CAD build for the part. Positions are in the model's coordinates, mm. Face numbers are marked on the shaded views. A direction names the side the tool comes from. Coordinates: 2 decimals unless noted, no trailing zeros. Order: outer loops, then holes, each group sorted by start corner. A loop starts at its lowest first (then second) coordinate and runs counter-clockwise, first axis right, second up. Notation, with made-up numbers: (55, 14) - (67, 14) arc R25 cw to (67, 35) - close; hole circle Ø4 at (51.5, 36.5). An arc over 180 degrees is marked (long way). Use one line per item in the form item = value.
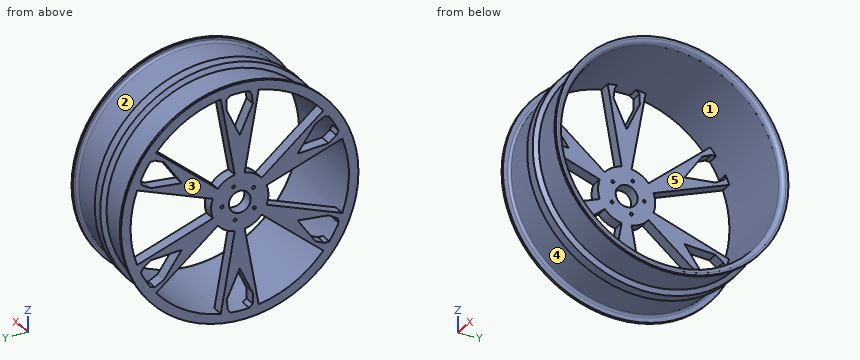
```python
from build123d import *

# Parameters (mm, degrees)
F2_R     = 3.1146523594
F2_R_2   = 22.9197931693
F3_DEPTH = 25
F4_COUNT = 6
F5_DEPTH = 25


# Not quite as in the source:
# - a feature names something its author has since deleted; it is built from what else it names


with BuildPart() as f1:
    # F0 (on Top) → F1 (revolve)
    with BuildSketch(Plane.XY):
        with BuildLine():
            Line((-79.7097083151, 53.5523933172), (-79.7097083151, 33.5523933172))
            Line((-79.7097083151, 33.5523933172), (113.4902916849, 33.5523933172))
            ThreePointArc((113.4902916849, 33.5523933172), (120.5613594967, 36.4813255054), (123.4902916849, 43.5523933172))
            Line((123.4902916849, 43.5523933172), (123.4902916849, 48.5523933172))
            Line((123.4902916849, 48.5523933172), (118.4902916849, 48.5523933172))
            Line((118.4902916849, 48.5523933172), (118.4902916849, 43.5523933172))
            ThreePointArc((118.4902916849, 43.5523933172), (117.0258255908, 40.0168594113), (113.4902916849, 38.5523933172))
            Line((113.4902916849, 38.5523933172), (38.4902916849, 38.5523933172))
            Line((38.4902916849, 38.5523933172), (5.2902916849, 38.5523933172))
            Line((5.2902916849, 38.5523933172), (-69.7097083151, 38.5523933172))
            ThreePointArc((-69.7097083151, 38.5523933172), (-73.2452422211, 40.0168594113), (-74.7097083151, 43.5523933172))
            Line((-74.7097083151, 43.5523933172), (-74.7097083151, 53.5523933172))
            Line((-74.7097083151, 53.5523933172), (-79.7097083151, 53.5523933172))
        make_face()
        Polygon((11.0637943768, 48.5523933172), (5.2902916849, 38.5523933172), (38.4902916849, 38.5523933172), (32.716788993, 48.5523933172), align=None)
    revolve(axis=Axis((21.8902916849, -195.0476066828, 0), (1, 0, 0)))

    # F2 (on face) → F3 (join)
    with BuildSketch(Plane(origin=(-79.7097083151, 0, 0), x_dir=(0, -1, 0), z_dir=(-1, 0, 0))):
        with BuildLine():
            ThreePointArc((184.6287160228, 59.0884651807), (189.8182621179, 59.7716818855), (195.0476066828, 60))
            Line((195.0476066828, 60), (195.0476066828, 139.9987626345))
            Line((195.0476066828, 139.9987626345), (167.5774196696, 198.9087687919))
            Line((167.5774196696, 198.9087687919), (167.7933331286, 221.202246743))
            Line((167.7933331286, 221.202246743), (175.3516332681, 227.7499256449))
            ThreePointArc((175.3516332681, 227.7499256449), (165.3226894728, 226.6591919532), (155.3516332681, 225.1270523386))
            Line((155.3516332681, 225.1270523386), (184.6287160228, 59.0884651807))
        make_face()
        with BuildLine():
            Line((195.0476066828, 139.9987626345), (195.0476066828, 60))
            ThreePointArc((195.0476066828, 60), (200.2769512476, 59.7716818855), (205.4664973428, 59.0884651807))
            Line((205.4664973428, 59.0884651807), (234.7435800974, 225.1270523386))
            ThreePointArc((234.7435800974, 225.1270523386), (224.7725238927, 226.6591919532), (214.7435800974, 227.7499256449))
            Line((214.7435800974, 227.7499256449), (220.1414219841, 219.3318912564))
            Line((220.1414219841, 219.3318912564), (222.5177936959, 198.9087687919))
            Line((222.5177936959, 198.9087687919), (195.0476066828, 139.9987626345))
        make_face()
        with BuildLine():
            ThreePointArc((205.4664973428, 59.0884651807), (200.2769512476, 59.7716818855), (195.0476066828, 60))
            ThreePointArc((195.0476066828, 60), (189.8182621179, 59.7716818855), (184.6287160228, 59.0884651807))
            ThreePointArc((184.6287160228, 59.0884651807), (156.4803501016, -45.9626665871), (255.0476066828, 0))
            ThreePointArc((255.0476066828, 0), (241.0102732699, 38.5672565812), (205.4664973428, 59.0884651807))
        make_face()
        with Locations((158.1552479456, -1.5052259386)):
            Circle(F2_R, mode=Mode.SUBTRACT)
        with Locations((185.0787958079, -35.5518585739)):
            Circle(F2_R, mode=Mode.SUBTRACT)
        with Locations((195.0476066828, 0)):
            Circle(F2_R_2, mode=Mode.SUBTRACT)
        with Locations((225.7789014718, -20.4670310233)):
            Circle(F2_R, mode=Mode.SUBTRACT)
        with Locations((224.0094022556, 22.9025377527)):
            Circle(F2_R, mode=Mode.SUBTRACT)
        with Locations((182.215685933, 34.6215777831)):
            Circle(F2_R, mode=Mode.SUBTRACT)
    extrude(amount=-F3_DEPTH)

    # F4: F1 ×6 about axis
    f4_axis = Axis((21.8902916849, -195.0476066828, 0), (1, 0, 0))


with BuildPart() as f1_1:
    add(f1.part)
    for i in range(1, F4_COUNT):
        add(f1.part.rotate(f4_axis, i * 360 / F4_COUNT))

    # F2 (on face) → F5 (cut)
    with BuildSketch(Plane(origin=(-79.7097083151, 0, 0), x_dir=(0, -1, 0), z_dir=(-1, 0, 0))):
        with Locations((158.1552479456, -1.5052259386)):
            Circle(F2_R)
        with Locations((182.215685933, 34.6215777831)):
            Circle(F2_R)
        with Locations((224.0094022556, 22.9025377527)):
            Circle(F2_R)
        with Locations((225.7789014718, -20.4670310233)):
            Circle(F2_R)
        with Locations((185.0787958079, -35.5518585739)):
            Circle(F2_R)
        with Locations((195.0476066828, 0)):
            Circle(F2_R_2)
    extrude(amount=-F5_DEPTH, mode=Mode.SUBTRACT)


solid = f1_1.part
```
Item 1: Cut at B-B, the plane z = 159.5. State how many separate pieces and enclosed holes the cut face has, plus the area to 3 significant figures.
Derived:
separate_pieces = 4
enclosed_holes = 0
area = 4,800 mm²
Item 2: Drop flat-ended pins along their axis: pin 1 (1 mm diameter, centred on y = -185, z = -109.5, fed in from +X); pin 2 (8 mm diameter, centred on x = -24.5, y = -238, fed in from -Z); pin 3 (5.5 mm diameter, centred on y = -158.16, z = -1.51, fed in from +X); pin 4 (2 mm diameter, centred on x = 14.5, y = 2, fed in from +Z). Give the stop position or say it passes through.
Derived:
pin_1 = -54.71
pin_2 = -230.33
pin_3 = through
pin_4 = 144.59
Item 3: Cut at A-A, the plane x = 61.5. Write the cut outline in (y, z), plus the area to 3 significant figures.
Derived:
outline = circle Ø467.2 at (-195.05, 0); hole circle Ø457.2 at (-195.05, 0)
area = 7,260 mm²
Item 4: Two-plate mould, pull along Z, no slides. Class the marked faces 1, 2 and 3: +Z half, -Z half, draft (parallel to the pull), parting line (faces both ways), or undercut.
Derived:
face_1 = undercut
face_2 = parting line
face_3 = draft
Item 5: 3-axis set-ups, long thin cutter, end or side, ignore diameter. For the marked faces 4 and 5: which of +Z, -Z, +X, -X, +Y, -Y reach the whole face in a straight line?
Derived:
face_4 = none
face_5 = +X
Item 6: Drill centre lines: line 1 (Y direction, x = -70.5, z = -168); line 2 (Z direction, x = 101, y = -167); line 3 (Y direction, x = -63.5, z = 136.5). Where is each one in solid material? Low to high. Write a range as [from, to].
Derived:
line_1 = [-357.45, -350.08], [-224.67, -208.1], [-181.99, -165.42], [-40.02, -32.65]
line_2 = [-231.91, -226.87], [226.87, 231.91]
line_3 = [-384.62, -357.72], [-219.12, -170.98], [-32.37, -5.48]
